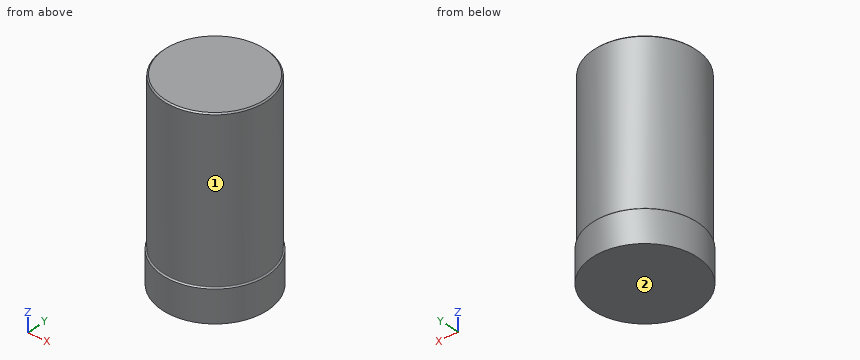
```python
from build123d import *

# Parameters (mm, degrees)
F0_R     = 6
F1_DEPTH = 22.5
F2_R     = 6.15
F3_DEPTH = 3.75
F4_R     = 0.14999
F5_SIZE2 = 0.15
F5_SIZE  = 0.15


# Not quite as in the source:
# - a fillet or chamfer is up to 0.001 mm smaller than in the source, because OpenCascade refuses the exact size


with BuildPart() as f1:
    # F0 (on Top) → F1 (new body)
    with BuildSketch(Plane.XY):
        Circle(F0_R)
    extrude(amount=F1_DEPTH)

    # F2 (on Top) → F3 (join)
    with BuildSketch(Plane.XY):
        Circle(F2_R)
    extrude(amount=F3_DEPTH)

    # F4 (radius 0.15 in the source; OpenCascade refuses exactly that, so slightly less here)
    f4_edges = [f1.edges().sort_by_distance(p)[0] for p in [
        (-6, 0, 3.75),
    ]]
    fillet(f4_edges, radius=F4_R)

    # F5
    f5_edges = [f1.edges().sort_by_distance(p)[0] for p in [
        (-6, 0, 22.5),
    ]]
    chamfer(f5_edges, length=F5_SIZE, length2=F5_SIZE2)


solid = f1.part
```
Geometry: final body of the model. Coordinates: model frame, mm. Face numbers are marked on the shaded views. A direction names the side the tool comes from. Round coordinates to 2 decimals unless told otherwise and drop trailing zeros. Order: outer loops, then holes, each group sorted by start corner. A loop starts at its lowest first (then second) coordinate and runs counter-clockwise, first axis right, second up. Notation, with made-up numbers: (-28, -33.75) -> (-11, -33.75) arc R23 cw to (-11, -19.75) -> close; hole circle Ø9 at (-3.75, 59.5). An arc over 180 degrees is marked (long way). Use CSV: the item, a comma, the result in double quotes. Start each with the question number.
1) Section C-C (z = 5.75). Return the cut outline in (x, y).
2) First-contact query: pin 1 Ø1 at (x, z) = (2.5, 7) entering from +Y; pin 2 Ø2 at (y, z) = (-4.5, 12.5) entering from +X; pin 3 Ø3 at (y, z) = (3.5, 3.5) entering from -X. Flat tips, straight axial feed; report the tip coordinate or a pass-through.
3) Set-up query: the marked faces 1 and 2. Return all of +Z, -Z, +X, -X, +Y, -Y with unobstructed straight access to the full face (end or side cutting, diameter ignored); none if empty.
4) Material intervals for line 1 along Y through (x, z) = (-4.75, 5.5); line 2 along X through (y, z) = (-4, 19.5); line 3 along Y through (x, z) = (5, 2), sorted ascending. Write a range as from..to.
Returned:
1,outline,"circle Ø12 at (0, 0)"
2,pin 1,"stops at y = 5.66"
2,pin 2,"stops at x = 4.87"
2,pin 3,"stops at x = -5.82"
3,face 1,"+Z"
3,face 2,"-Z, +X, -X, +Y, -Y"
4,line 1,"y = -3.67..3.67"
4,line 2,"x = -4.47..4.47"
4,line 3,"y = -3.58..3.58"
